The model under review builds one solid part; all positions refer to its coordinate system, in mm. Face numbers are marked on the shaded views. A direction names the side the tool comes from. Round coordinates to 2 decimals unless told otherwise and drop trailing zeros. Write each loop counter-clockwise with the first axis right and the second up, starting at its lowest first coordinate (ties: lowest second). Pieces come first, ordered by that corner, then holes. Notation, with made-up numbers: (89.5, -25) -> (128.5, -25) arc R19 ccw to (128.5, -18) -> close; hole circle Ø8 at (56, -39.75). An arc over 180 degrees is marked (long way). Answer as a JSON object with one key per item and string values. Group by question number.
1) Insertion check: pin 1 Ø2 at (y, z) = (-3, 3) entering from -X; pin 2 Ø1.5 at (y, z) = (3.5, 2.5) entering from -X; pin 3 Ø3 at (x, z) = (2, 4.5) entering from +Y. Each pin has a flat end and moves straight along its axis. Give the tip position at first contact, or say it passes through.
2) We need section A-A, the plane z = 2. Write out the cut boundary in (x, y), then the cut area to 3 significant figures.
3) Machinability: for the marked faces 1 and 2, which of the approach directions +Z, -Z, +X, -X, +Y, -Y give a long, thin tool a straight path to every point of the face, cutting with its end or side? Answer none if there is none.
4) We need section C-C, the plane x = 4.5. Write out the cut boundary in (y, z).
5) We need section B-B, the plane y = 0. Write out the cut boundary in (x, z), then the cut area to 4 significant figures.
6) To check wall thickness, follow probe 1 along Z at (x, y) = (3.75, -5); probe 2 along X at (y, z) = (-2.5, 8.75); probe 3 along X at (y, z) = (-5, 3). State the ranges of each line that lie inside material, in increasing order. Write a range as [from, to].
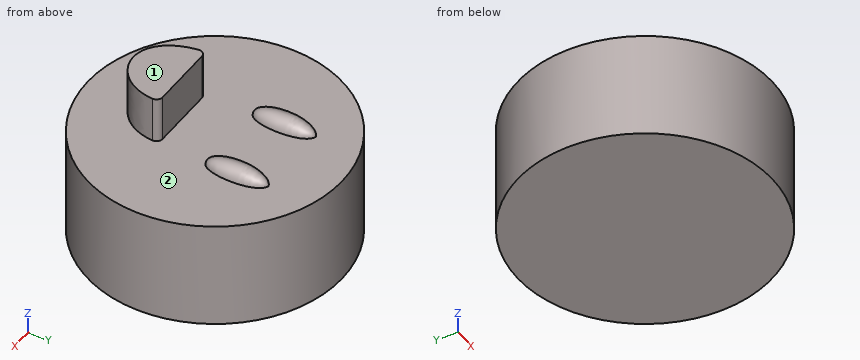
from build123d import *

# Parameters (mm, degrees)
F0_R     = 8.25
F1_DEPTH = 7
F5_DEPTH = 3


with BuildPart() as f1:
    # F0 (on Top) → F1 (new body)
    with BuildSketch(Plane.XY):
        Circle(F0_R)
    extrude(amount=F1_DEPTH)

    # F2 (on face) → F3 (revolve)
    with BuildSketch(Plane.XY.offset(7)):
        with BuildLine():
            Line((-2.5, 1), (-2.5, 5))
            add(Edge.make_bspline(
                [(-2.5, 1), (-3.43300635, 0.8503383724), (-3.585588187, 4.7030341811), (-2.5, 5)],
                knots=[0, 0, 0, 0, 4, 4, 4, 4], degree=3))
        make_face()
    revolve(axis=Axis((-2.5, 3, 7), (0, -1, 0)))

    # F2 (on face) → F4 (revolve)
    with BuildSketch(Plane.XY.offset(7)):
        with BuildLine():
            Line((2.5, 1), (2.5, 5))
            add(Edge.make_bspline(
                [(2.5, 1), (1.56699365, 0.8503383724), (1.414411813, 4.7030341811), (2.5, 5)],
                knots=[0, 0, 0, 0, 4, 4, 4, 4], degree=3))
        make_face()
    revolve(axis=Axis((2.5, 3, 7), (0, -1, 0)))

    # F2 (on face) → F5 (join)
    with BuildSketch(Plane.XY.offset(7)):
        with BuildLine():
            Line((2.0776409017, -2.1250108257), (-2.0717297527, -2.1250108257))
            ThreePointArc((-2.0717297527, -2.1250108257), (-2.374725272, -2.2638715616), (-2.4673498875, -2.5840422494))
            add(Edge.make_bspline(
                [(-2.4673498875, -2.5840422494), (-2.1958217419, -4.4037849366), (-0.0853140585, -6.3108429823), (2.3625802937, -4.2915575872), (2.4767824749, -2.5512025144)],
                knots=[0.0375043401, 0.0375043401, 0.0375043401, 0.0375043401, 0.50066272, 0.963428104, 0.963428104, 0.963428104, 0.963428104], degree=3))
            ThreePointArc((2.4767824749, -2.5512025144), (2.3695969562, -2.2515850364), (2.0776409017, -2.1250108257))
        make_face()
    extrude(amount=F5_DEPTH)


solid = f1.part
Here are the results:
{
 "1": {"pin 1": "stops at x = -8", "pin 2": "stops at x = -7.78", "pin 3": "stops at y = 8.23"},
 "2": {"outline": "circle Ø16.5 at (0, 0)", "area": "214 mm^2"},
 "3": {"face 1": "+Z, +X, -X, +Y, -Y", "face 2": "+Z"},
 "4": {"outline": "(-6.91, 0) -> (6.91, 0) -> (6.91, 7) -> (-6.91, 7) -> close"},
 "5": {"outline": "(-8.25, 0) -> (8.25, 0) -> (8.25, 7) -> (-8.25, 7) -> close", "area": "115.5 mm^2"},
 "6": {"probe 1": "z = [0, 7]", "probe 2": "x = [-2.47, 2.48]", "probe 3": "x = [-6.56, 6.56]"}
}
